Design review of the part built by this model. Coordinates are the model's own, in mm. A direction names the side the tool comes from. Coordinates: 2 decimals unless noted, no trailing zeros. Write each loop counter-clockwise with the first axis right and the second up, starting at its lowest first coordinate (ties: lowest second). Pieces come first, ordered by that corner, then holes. Notation, with made-up numbers: M 40.5,-32.75 L 60.5,-32.75 A30 cw 60.5,-9.75 Z; hole C 57,78.5 d11. An arc over 180 degrees is marked long. Return JSON: item names as keys, results as strings. Group by question number.
```python
from build123d import *

# Parameters (mm, degrees)
EXTRUDE_1_DEPTH = 38.1


with BuildPart() as part:
    # Эскиз1 → Бобышка-Вытянуть1 (new body)
    with BuildSketch(Plane.XY):
        with BuildLine():
            ThreePointArc((58.039129224, 77.945655108), (56.901327597, 79.116004883), (55.683853915, 80.203234837))
            ThreePointArc((55.683853915, 80.203234837), (29.318529457, 95.307848832), (-0.611231214, 100.550855968))
            ThreePointArc((-0.611231214, 100.550855968), (-15.584507099, 99.552637576), (-30.292769251, 96.575649981))
            ThreePointArc((-30.292769251, 96.575649981), (-33.129887493, 94.929167254), (-34.776370221, 92.092049011))
            ThreePointArc((-34.776370221, 92.092049011), (-38.751576208, 62.410510975), (-34.776370221, 32.728972938))
            ThreePointArc((-34.776370221, 32.728972938), (-33.129887493, 29.891854696), (-30.29276925, 28.245371968))
            ThreePointArc((-30.29276925, 28.245371968), (-15.584507098, 25.268384374), (-0.611231214, 24.270165982))
            ThreePointArc((-0.611231214, 24.270165982), (29.318529457, 29.513173118), (55.683853915, 44.617787113))
            ThreePointArc((55.683853915, 44.617787113), (56.901327595, 45.705017068), (58.039129224, 46.875366842))
            ThreePointArc((58.039129224, 46.875366842), (64.442309074, 62.410510975), (58.039129224, 77.945655108))
        make_face()
        with BuildLine():
            ThreePointArc((57.313391253, 77.25728346), (63.442309074, 62.410510975), (57.313391253, 47.56373849))
            ThreePointArc((57.313391253, 47.56373849), (56.217638563, 46.434884922), (55.04449071, 45.386691978))
            ThreePointArc((55.04449071, 45.386691978), (28.978606573, 30.453626431), (-0.611231214, 25.270165982))
            ThreePointArc((-0.611231214, 25.270165982), (-15.451763735, 26.259534816), (-30.029631964, 29.210130367))
            ThreePointArc((-30.029631964, 29.210130367), (-32.422780711, 30.598961477), (-33.811611821, 32.992110224))
            ThreePointArc((-33.811611821, 32.992110224), (-37.751576208, 62.410510974), (-33.811611822, 91.828911725))
            ThreePointArc((-33.811611822, 91.828911725), (-32.422780712, 94.222060472), (-30.029631965, 95.610891582))
            ThreePointArc((-30.029631965, 95.610891582), (-15.451763736, 98.561487134), (-0.611231214, 99.550855968))
            ThreePointArc((-0.611231214, 99.550855968), (28.978606573, 94.367395519), (55.04449071, 79.434329972))
            ThreePointArc((55.04449071, 79.434329972), (56.217638563, 78.386137027), (57.313391253, 77.25728346))
        make_face(mode=Mode.SUBTRACT)
    extrude(amount=EXTRUDE_1_DEPTH)


solid = part.part
```
Item 1: Add section C-C (y = 49). Write out the cut boundary in (x, z), plus the area to 3 significant figures.
Item 2: Add section A-A (z = 34.5). Write out the cut boundary in (x, y), plus the area to 3 significant figures.
Item 3: Add section B-B (x = -3.5). Write out the cut boundary in (y, z).
Item 4: For line 1 (X direction, y = 36, z = 21); line 2 (Y direction, x = 20, z = 17); line 3 (Y direction, x = -7, z = 22.5), list the stretches that pass through material, from the lowest coordinate up.
Item 5: The part is to be moulded in two halves that separate along Y. For faces 1 (the cylindrical face through (-15.38, 99.58, 18.78)), 2 (the flat face through (8.8, 99.3, 38.1)), 3 (the cylindrical face through (28.92, 29.37, 18.78)), 4 (the cylindrical face through (29.38, 30.6, 18.78)), say which applies: pulls with the +Y half, pulls with the -Y half, needs draft (parallel to the pull), parting line crosses it, or undercut.
Item 6: Machinability: for faces 5 (the cylindrical face through (-32.395, 30.571, 18.783)), 6 (the cylindrical face through (-38.75, 62.83, 18.78)), which of the approach directions +Z, -Z, +X, -X, +Y, -Y give a long, thin tool a straight path to every point of the face, cutting with its end or side? Answer none if there is none.
Item 7: For pin 1 (1.5 mm diameter, centred on x = 41.5, z = 31, fed in from -Y); pin 2 (5 mm diameter, centred on x = -18.5, z = 24.5, fed in from -Y); pin 3 (2 mm diameter, centred on x = -22, z = 10, fed in from -Y), all flat-tipped, find the tip position at first contact; note any pin that passes through.
Geometry check:
{
 "1": {"outline": "M -37.95,0 L -36.94,0 L -36.94,38.1 L -37.95,38.1 Z; M 58.62,0 L 59.89,0 L 59.89,38.1 L 58.62,38.1 Z", "area": "87.1 mm^2"},
 "2": {"outline": "M -34.78,32.73 A6.39 ccw -30.29,28.25 A112.8 ccw -0.61,24.27 A88.05 ccw 55.68,44.62 A23.14 ccw 58.04,46.88 A22.05 ccw 58.04,77.95 A23.14 ccw 55.68,80.2 A88.05 ccw -0.61,100.55 A112.8 ccw -30.29,96.58 A6.39 ccw -34.78,92.09 A112.8 ccw Z; hole M -33.81,32.99 A5.39 ccw -30.03,29.21 A111.8 ccw -0.61,25.27 A87.05 ccw 55.04,45.39 A22.14 ccw 57.31,47.56 A21.05 ccw 57.31,77.26 A22.14 ccw 55.04,79.43 A87.05 ccw -0.61,99.55 A111.8 ccw -30.03,95.61 A5.39 ccw -33.81,91.83 A111.8 ccw Z", "area": "293 mm^2"},
 "3": {"outline": "M 24.31,0 L 25.31,0 L 25.31,38.1 L 24.31,38.1 Z; M 99.51,0 L 100.51,0 L 100.51,38.1 L 99.51,38.1 Z"},
 "4": {"line 1": "-35.62 to -34.59, 41.26 to 43.3", "line 2": "26.72 to 27.75, 97.08 to 98.1", "line 3": "24.45 to 25.45, 99.37 to 100.37"},
 "5": {"face 1": "pulls with the +Y half", "face 2": "needs draft", "face 3": "pulls with the -Y half", "face 4": "undercut"},
 "6": {"face 5": "+Z, -Z", "face 6": "+Z, -Z, -X"},
 "7": {"pin 1": "y = 34.59", "pin 2": "y = 25.32", "pin 3": "y = 26.13"}
}
